Geometry check sheet. Reference: the model listing, model coordinates, mm. A direction names the side the tool comes from. Round coordinates to 2 decimals unless told otherwise and drop trailing zeros. Order: outer loops, then holes, each group sorted by start corner. A loop starts at its lowest first (then second) coordinate and runs counter-clockwise, first axis right, second up.
```python
from build123d import *

# Parameters (mm, degrees)
F0_W     = 48
F0_H     = 26
F0_R     = 1.5
F0_R_2   = 1.6
F1_DEPTH = 2
F2_W     = 25
F2_H     = 18
F3_DEPTH = 15
F5_DEPTH = 25


with BuildPart() as f1:
    # F0 (on Top) → F1 (new body)
    with BuildSketch(Plane.XY):
        Rectangle(F0_W, F0_H)
        with Locations((-21.5, -9.5)):
            Circle(F0_R, mode=Mode.SUBTRACT)
        with Locations((21.5, -9.5)):
            Circle(F0_R, mode=Mode.SUBTRACT)
        with Locations((-16.5, 0)):
            Circle(F0_R_2, mode=Mode.SUBTRACT)
        with Locations((-21.5, 8.9)):
            Circle(F0_R, mode=Mode.SUBTRACT)
        with Locations((16.5, 0)):
            Circle(F0_R_2, mode=Mode.SUBTRACT)
        with Locations((21.5, 8.9)):
            Circle(F0_R, mode=Mode.SUBTRACT)
    extrude(amount=F1_DEPTH)

    # F2 (on face) → F3 (join)
    with BuildSketch(Plane.XY.offset(2)):
        Rectangle(F2_W, F2_H)
    extrude(amount=F3_DEPTH)

    # F4 (on face) → F5 (cut)
    with BuildSketch(Plane(origin=(-12.5, 0, 0), x_dir=(0, -1, 0), z_dir=(-1, 0, 0))):
        Polygon((-9, 17), (-9, 2), (0, 17), align=None)
        Polygon((9, 17), (0, 17), (9, 2), align=None)
    extrude(amount=-F5_DEPTH, mode=Mode.SUBTRACT)


solid = f1.part
```
(1) Sectioned sample at A-A, the plane x = -16.5. Record the cut outline in (y, z), and give its area (3 significant figures).
Returned:
outline: (-13, 0) - (-1.6, 0) - (-1.6, 2) - (-13, 2) - close; (1.6, 0) - (13, 0) - (13, 2) - (1.6, 2) - close
area: 45.6 mm2
(2) Draft check along Y on faces 6 (the cylindrical face through (20, 8.97, 0.99)), 7 (the flat face through (24, 0, 1)), 8 (the flat face through (0, -13, 1)). Enter one of: released by +Y, released by -Y, zero draft, split by the parting line, or undercut.
Returned:
face 6: undercut
face 7: zero draft
face 8: released by -Y
(3) Material ranges on line 1 (Y direction, x = 21.5, z = 1.5); line 2 (X direction, y = 0, z = 4.5); line 3 (Z direction, x = 15, y = -6), recorded low to high.
Returned:
line 1: y = -13 to -11, -8 to 7.4, 10.4 to 13
line 2: x = -12.5 to 12.5
line 3: z = 0 to 2
(4) Depth check by flat-ended pin: P1, Ø5, axis at y = -6.5, z = 10.5, coming from the -X side; P2, Ø5, axis at x = -21.5, y = 8.9, coming from the +Z side; P3, Ø5, axis at x = -21.5, y = -9.5, coming from the -Z side. Enter the tip coordinate at first touch or a pass-through.
Returned:
P1: stops at x = -12.5
P2: stops at z = 2
P3: stops at z = 0
(5) Sectioned sample at D-D, the plane z = 8.25. Record the cut outline in (x, y), and give its area (4 significant figures).
Returned:
outline: (-12.5, -5.25) - (12.5, -5.25) - (12.5, 5.25) - (-12.5, 5.25) - close
area: 262.5 mm2
(6) Set-up check for faces 1 (the flat face through (-0.18, 4.56, 9.4)), 2 (the flat face through (0, -11, 2)), 3 (the cylindrical face through (-18.1, 0.07, 0.99)), 4 (the flat face through (12.5, 0, 8)), 5 (the flat face through (-12.5, 0, 8)): record each of +Z, -Z, +X, -X, +Y, -Y from which the full face is reachable in a straight line by a thin tool's end or side.
Returned:
face 1: +Z, +X, -X, +Y
face 2: +Z
face 3: +Z, -Z
face 4: +Z, +X, +Y, -Y
face 5: +Z, -X, +Y, -Y
(7) Sectioned sample at C-C, the plane x = -21.5. Record the cut outline in (y, z).
Returned:
outline: (-13, 0) - (-11, 0) - (-11, 2) - (-13, 2) - close; (-8, 0) - (7.4, 0) - (7.4, 2) - (-8, 2) - close; (10.4, 0) - (13, 0) - (13, 2) - (10.4, 2) - close
(8) Sectioned sample at B-B, the plane y = -9.5. Record the cut outline in (x, z), and give its area (3 significant figures).
Returned:
outline: (-24, 0) - (-23, 0) - (-23, 2) - (-24, 2) - close; (-20, 0) - (20, 0) - (20, 2) - (-20, 2) - close; (23, 0) - (24, 0) - (24, 2) - (23, 2) - close
area: 84.0 mm2
